Could you check a few things on this drawing? It's one solid part, dimensions in mm from its lowest x, y, z. Round coordinates to 2 decimals unless told otherwise and drop trailing zeros. Loops run counter-clockwise (first coordinate to the right, second up) from the corner with the lowest first, then second, coordinate; pieces in that order, holes last. Notation, with made-up numbers: M -26.5,41 L 6.5,41 A8 ccw 6.5,47 Z; hole C 4.5,54.5 d10. An arc over 180 degrees is marked long. Answer as CSV lines item,"result".
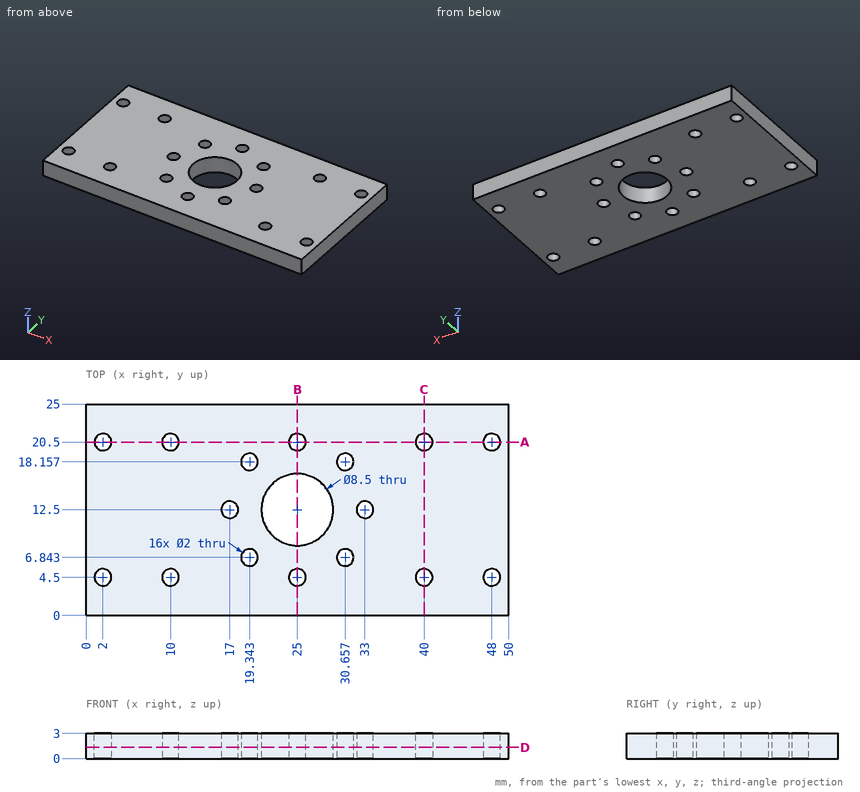
Item 1: If we section it at B-B on x = 25: Write out the boundary of the cut face in (y, z).
Output:
outline,"M 0,0 L 3.5,0 L 3.5,3 L 0,3 Z; M 5.5,0 L 8.25,0 L 8.25,3 L 5.5,3 Z; M 16.75,0 L 19.5,0 L 19.5,3 L 16.75,3 Z; M 21.5,0 L 25,0 L 25,3 L 21.5,3 Z"
Item 2: If we section it at D-D on z = 1.35: State how many separate pieces and enclosed holes the cut face has, then the cut area to 3 significant figures.
Output:
separate pieces,"1"
enclosed holes,"17"
area,"1,140 mm2"
Item 3: If I drill on line 1 along X through (y, z) = (6, 2.4) (1 decimal); line 2 along X through (y, z) = (4, 0.5); line 3 along X through (y, z) = (7, 2.45), over which ranges is the centre line in solid material (lowest first)? Write a range as from..to.
Output:
line 1,"x = 0..18.8, 19.9..30.1, 31.2..50"
line 2,"x = 0..1.13, 2.87..9.13, 10.87..24.13, 25.87..39.13, 40.87..47.13, 48.87..50"
line 3,"x = 0..18.36, 20.33..29.67, 31.64..50"
Item 4: If we section it at C-C on x = 40: Write out the boundary of the cut face in (y, z).
Output:
outline,"M 0,0 L 3.5,0 L 3.5,3 L 0,3 Z; M 5.5,0 L 19.5,0 L 19.5,3 L 5.5,3 Z; M 21.5,0 L 25,0 L 25,3 L 21.5,3 Z"
Item 5: If we section it at A-A on y = 20.5: Write out the boundary of the cut face in (x, z).
Output:
outline,"M 0,0 L 1,0 L 1,3 L 0,3 Z; M 3,0 L 9,0 L 9,3 L 3,3 Z; M 11,0 L 24,0 L 24,3 L 11,3 Z; M 26,0 L 39,0 L 39,3 L 26,3 Z; M 41,0 L 47,0 L 47,3 L 41,3 Z; M 49,0 L 50,0 L 50,3 L 49,3 Z"
